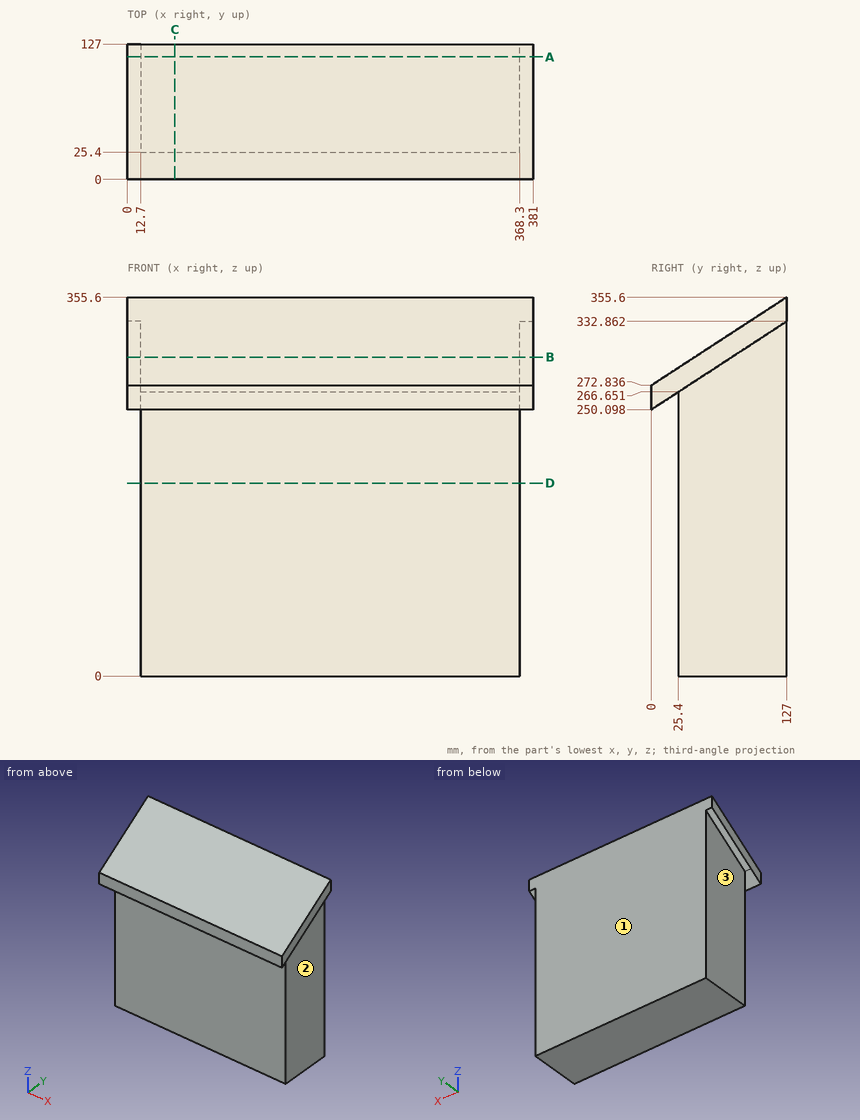
Geometry check sheet. Reference: drawing and pictorial views, mm from the part's lowest x, y, z. A direction names the side the tool comes from. Round coordinates to 2 decimals unless told otherwise and drop trailing zeros. Loops run counter-clockwise (first coordinate to the right, second up) from the corner with the lowest first, then second, coordinate; pieces in that order, holes last. Notation, with made-up numbers: (81, 64) - (103, 64) arc R24 ccw to (103, 81) - close; hole circle Ø2 at (30, 44). An arc over 180 degrees is marked (long way). One line per question, with ' | ' between items. Start each with the question number.
1. Cross-section at D-D on z = 181. Record the cut outline in (x, y).
2. Cross-section at B-B on z = 299.5. Record the cut outline in (x, y) (1 decimal), then the cut area to 3 significant figures.
3. Depth check by flat-ended pin: pin 1 (8 mm diameter, centred on y = 38.5, z = 229.5, fed in from -X); pin 2 (1.5 mm diameter, centred on y = 30, z = 137, fed in from +X); pin 3 (2 mm diameter, centred on x = 321.5, z = 194, fed in from -Y); pin 4 (1.5 mm diameter, centred on x = 218.5, y = 75, fed in from -Z). Enter the tip coordinate at first touch or a pass-through.
4. Tool access check on the marked faces 1, 2 and 3. Record the directions out of +Z, -Z, +X, -X, +Y, -Y that give a thin tool (end or side, any length) a straight path to the whole face; none if there is none.
5. Cross-section at C-C on x = 44.5. Record the cut outline in (y, z), then the cut area to 3 significant figures.
6. Scan lines: line 1 (Y direction, x = 319.5, z = 35); line 2 (X direction, y = 27, z = 145.5); line 3 (Z direction, x = 126.5, y = 107) (1 decimal). Record each from-to range of solid material in increasing order. Write a range as [from, to].
7. Cross-section at A-A on y = 115. Record the cut outline in (x, z), then the cut area to 3 significant figures.
Taken from the geometry:
1) outline: (12.7, 25.4) - (368.3, 25.4) - (368.3, 127) - (12.7, 127) - close
2) outline: (0, 40.9) - (381, 40.9) - (381, 75.8) - (368.3, 75.8) - (368.3, 127) - (12.7, 127) - (12.7, 75.8) - (0, 75.8) - close | area: 31,500 mm²
3) pin 1: x = 12.7 | pin 2: x = 368.3 | pin 3: y = 25.4 | pin 4: z = 0
4) face 1: +Z, -Z, +X, -X, +Y | face 2: -Z, +X, +Y | face 3: -Z, -X, +Y
5) outline: (0, 250.1) - (25.4, 266.65) - (25.4, 0) - (127, 0) - (127, 355.6) - (0, 272.84) - close | area: 33,300 mm²
6) line 1: [25.4, 127] | line 2: [12.7, 368.3] | line 3: [0, 342.6]
7) outline: (0, 325.04) - (12.7, 325.04) - (12.7, 0) - (368.3, 0) - (368.3, 325.04) - (381, 325.04) - (381, 347.78) - (0, 347.78) - close | area: 124,000 mm²
